Check sheet for the modelled part. Datum: model origin and axes. Units: mm. A direction names the side the tool comes from. Round coordinates to 2 decimals unless told otherwise and drop trailing zeros. Order: outer loops, then holes, each group sorted by start corner. A loop starts at its lowest first (then second) coordinate and runs counter-clockwise, first axis right, second up.
Q1. Mould release check, pull along Z, two halves, no side actions. Record for faces 1 (the flat face through (17, 10, -13)), 2 (the flat face through (18, 2, -14)), 3 (the flat face through (0, 1, 30)): +Z half, -Z half, draft (parallel to the pull), parting line (faces both ways), or undercut.
Q2. Cross-section at D-D on y = 1. Record the cut outline in (x, z).
Q3. Cross-section at C-C on x = 11.5. Record the cut outline in (y, z).
Q4. Set-up check for faces 4 (the cylindrical face through (-17.49, 5.94, 13.14)), 5 (the flat face through (0, 0, 0)), 6 (the flat face through (0, 1, 26.75)): record each of +Z, -Z, +X, -X, +Y, -Y from which the full face is reachable in a straight line by a thin tool's end or side.
Q5. Cross-section at B-B on z = 25. Record the cut outline in (x, y).
Q6. Cross-section at A-A on y = 7. Record the cut outline in (x, z), then the cut area to 3 significant figures.
Q7. Depth check by flat-ended pin: P1, Ø3.5, axis at x = -18.5, z = 14.25, coming from the -Y side; P2, Ø1.5, axis at x = 18, z = -14, coming from the +Y side; P3, Ø4, axis at y = 9, z = -18.5, coming from the -X side. Enter the tip coordinate at first touch or a pass-through.
Q8. Scan lines: probe 1 along X at (y, z) = (6, -14.25); probe 2 along Y at (x, z) = (-11.5, -19). Record each from-to range of solid material in increasing order.
from build123d import *

# Parameters (mm, degrees)
SKETCH1_W           = 47
SKETCH1_H           = 60
BOSS_EXTRUDE1_DEPTH = 2
SKETCH2_R           = 2.7
SKETCH2_R_2         = 1.5
BOSS_EXTRUDE2_DEPTH = 8


with BuildPart() as part:
    # Sketch1 → Boss-Extrude1 (new body)
    with BuildSketch(Plane(origin=(0, 0, 0), x_dir=(1, 0, 0), z_dir=(0, 1, 0))):
        Rectangle(SKETCH1_W, SKETCH1_H)
        with BuildLine():
            Line((-17.98240987, 26.75), (17.98240987, 26.75))
            ThreePointArc((17.98240987, 26.75), (19.73240987, 25), (17.98240987, 23.25))
            Line((17.98240987, 23.25), (-17.98240987, 23.25))
            ThreePointArc((-17.98240987, 23.25), (-19.73240987, 25), (-17.98240987, 26.75))
        make_face(mode=Mode.SUBTRACT)
        with BuildLine():
            Line((-17.98240987, -23.25), (17.98240987, -23.25))
            ThreePointArc((17.98240987, -23.25), (19.73240987, -25), (17.98240987, -26.75))
            Line((17.98240987, -26.75), (-17.98240987, -26.75))
            ThreePointArc((-17.98240987, -26.75), (-19.73240987, -25), (-17.98240987, -23.25))
        make_face(mode=Mode.SUBTRACT)
    extrude(amount=BOSS_EXTRUDE1_DEPTH)

    # Sketch2 → Boss-Extrude2 (add)
    # profile 1 of 4: a face of its own
    with BuildSketch(Plane(origin=(0, 2, 0), x_dir=(1, 0, 0), z_dir=(0, 1, 0))):
        with Locations(Location((-18.5, 14.25, 0), (0, 0, 270))):
            Circle(SKETCH2_R)
        with Locations(Location((-18.5, 14.25, 0), (0, 0, 270))):
            Circle(SKETCH2_R_2, mode=Mode.SUBTRACT)
    # profile 2 of 4: a face of its own
    with BuildSketch(Plane(origin=(0, 2, 0), x_dir=(1, 0, 0), z_dir=(0, 1, 0))):
        with Locations(Location((18.5, 14.25, 0), (0, 0, 270))):
            Circle(SKETCH2_R)
        with Locations(Location((18.5, 14.25, 0), (0, 0, 270))):
            Circle(SKETCH2_R_2, mode=Mode.SUBTRACT)
    # profile 3 of 4: a face of its own
    with BuildSketch(Plane(origin=(0, 2, 0), x_dir=(1, 0, 0), z_dir=(0, 1, 0))):
        with Locations(Location((18.5, -14.25, 0), (0, 0, 270))):
            Circle(SKETCH2_R)
        with Locations(Location((18.5, -14.25, 0), (0, 0, 270))):
            Circle(SKETCH2_R_2, mode=Mode.SUBTRACT)
    # profile 4 of 4: a face of its own
    with BuildSketch(Plane(origin=(0, 2, 0), x_dir=(1, 0, 0), z_dir=(0, 1, 0))):
        with Locations(Location((-18.5, -14.25, 0), (0, 0, 270))):
            Circle(SKETCH2_R)
        with Locations(Location((-18.5, -14.25, 0), (0, 0, 270))):
            Circle(SKETCH2_R_2, mode=Mode.SUBTRACT)
    extrude(amount=BOSS_EXTRUDE2_DEPTH)


solid = part.part
Results found:
1. face 1: draft
1. face 2: undercut
1. face 3: +Z half
2. outline: (-23.5, -30) - (23.5, -30) - (23.5, 30) - (-23.5, 30) - close; hole (-17.98, -26.75) - (17.98, -26.75) arc R1.75 ccw to (17.98, -23.25) - (-17.98, -23.25) arc R1.75 ccw to start; hole (-17.98, 23.25) - (17.98, 23.25) arc R1.75 ccw to (17.98, 26.75) - (-17.98, 26.75) arc R1.75 ccw to start
3. outline: (0, -30) - (2, -30) - (2, -26.75) - (0, -26.75) - close; (0, -23.25) - (2, -23.25) - (2, 23.25) - (0, 23.25) - close; (0, 26.75) - (2, 26.75) - (2, 30) - (0, 30) - close
4. face 4: +Y
4. face 5: +Z, -Z, +X, -X, -Y
4. face 6: +Y, -Y
5. outline: (-23.5, 0) - (-19.73, 0) - (-19.73, 2) - (-23.5, 2) - close; (19.73, 0) - (23.5, 0) - (23.5, 2) - (19.73, 2) - close
6. outline: circle Ø5.4 at (-18.5, -14.25); circle Ø5.4 at (-18.5, 14.25); circle Ø5.4 at (18.5, -14.25); circle Ø5.4 at (18.5, 14.25); hole circle Ø3 at (-18.5, -14.25); hole circle Ø3 at (-18.5, 14.25); hole circle Ø3 at (18.5, -14.25); hole circle Ø3 at (18.5, 14.25)
6. area: 63.3 mm2
7. P1: stops at y = 0
7. P2: stops at y = 2
7. P3: stops at x = -19.99
8. probe 1: x = -21.2 to -20, -17 to -15.8, 15.8 to 17, 20 to 21.2
8. probe 2: y = 0 to 2
